from build123d import *

# Parameters (mm, degrees)
EXTRUDE_THIN1_DEPTH = 30
SKETCH2_R           = 4.1
CUT_EXTRUDE1_DEPTH  = 10
BOSS_EXTRUDE1_START = -3
SKETCH3_W           = 40
SKETCH3_H           = 40
BOSS_EXTRUDE1_DEPTH = 15
SKETCH4_R           = 6
BOSS_EXTRUDE2_DEPTH = 5
FILLET1_R           = 2
SKETCH5_W           = 40
SKETCH5_H           = 40
SKETCH5_W_2         = 38
SKETCH5_H_2         = 38
BOSS_EXTRUDE3_DEPTH = 40
SKETCH6_W           = 40
SKETCH6_H           = 40
BOSS_EXTRUDE4_DEPTH = 1
SKETCH7_R           = 2.5
CUT_EXTRUDE2_DEPTH  = 91.691785736


with BuildPart() as part:
    # Sketch1 → Extrude-Thin1 (new body)
    with BuildSketch(Plane(origin=(0, 0, 0), x_dir=(1, 0, 0), z_dir=(0, 1, 0))):
        Polygon((0, 0), (60, 0), (60, -15), (57, -15), (57, -3), (0, -3), align=None)
    extrude(amount=EXTRUDE_THIN1_DEPTH)

    # Sketch2 → Cut-Extrude1 (cut)
    with BuildSketch(Plane.XY.offset(3)):
        with Locations((15, 15)):
            Circle(SKETCH2_R)
    extrude(amount=-CUT_EXTRUDE1_DEPTH, mode=Mode.SUBTRACT)

    # Sketch3 → Boss-Extrude1 (add)
    with BuildSketch(Plane.ZY.offset(-57).offset(BOSS_EXTRUDE1_START)):
        with Locations((35, 20)):
            Rectangle(SKETCH3_W, SKETCH3_H)
    extrude(amount=BOSS_EXTRUDE1_DEPTH)

    # Sketch4 → Boss-Extrude2 (add)
    with BuildSketch(Plane.ZY.offset(-45)):
        with Locations(Location((35, 20, 0), (0, 0, 180))):
            Circle(SKETCH4_R)
    extrude(amount=BOSS_EXTRUDE2_DEPTH)

    # Fillet1
    fillet1_edges = [part.edges().sort_by_distance(p)[0] for p in [
        (45, 20, 41),
    ]]
    fillet(fillet1_edges, radius=FILLET1_R)

    # Sketch5 → Boss-Extrude3 (add)
    with BuildSketch(Plane.ZY.offset(-45)):
        with Locations((35, 20)):
            Rectangle(SKETCH5_W, SKETCH5_H)
        with Locations((35, 20)):
            Rectangle(SKETCH5_W_2, SKETCH5_H_2, mode=Mode.SUBTRACT)
    extrude(amount=BOSS_EXTRUDE3_DEPTH)

    # Sketch6 → Boss-Extrude4 (add)
    with BuildSketch(Plane.ZY.offset(-5)):
        with Locations((35, 20)):
            Rectangle(SKETCH6_W, SKETCH6_H)
    extrude(amount=BOSS_EXTRUDE4_DEPTH)

    # Sketch7 → Cut-Extrude2 (cut, through all)
    with BuildSketch(Plane(origin=(0, 40, 0), x_dir=(1, 0, 0), z_dir=(0, 1, 0))):
        with Locations(Location((15, -35, 0), (0, 0, 270))):
            Circle(SKETCH7_R)
    extrude(amount=-CUT_EXTRUDE2_DEPTH, mode=Mode.SUBTRACT)

    # Sketch8 → Revolve1 (revolve)
    with BuildSketch(Plane.XY.offset(35), mode=Mode.PRIVATE) as revolve1_sk:
        Polygon((17.5, 1), (22.966741001, 8.14945752), (23.966741001, 8.14945752), (23.966741001, 1), align=None)
    revolve(revolve1_sk.sketch.rotate(Axis((15, 1, 35), (0, 1, 0)), 90), axis=Axis((15, 1, 35), (0, 1, 0)))


solid = part.part
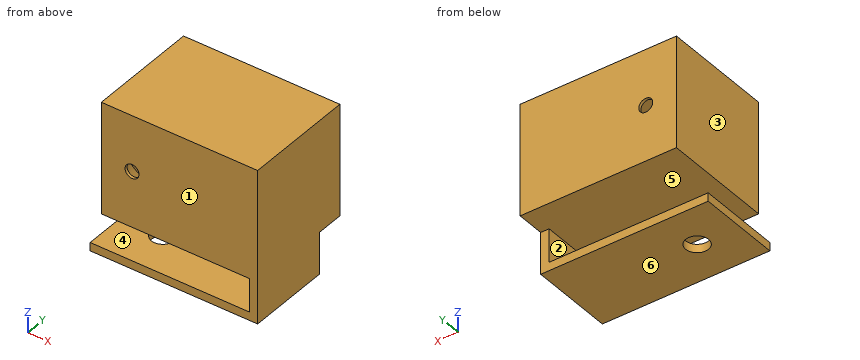
The listing builds one solid part. Answer for the finished solid, in the listing's coordinates (mm). Face numbers are marked on the shaded views. A direction names the side the tool comes from. Give positions to 0.01 mm unless a question says otherwise; leave off trailing zeros. Loops run counter-clockwise (first coordinate to the right, second up) from the corner with the lowest first, then second, coordinate; pieces in that order, holes last. Notation, with made-up numbers: (14.5, -23.5) - (52.5, -23.5) arc R28 ccw to (52.5, 1.5) - close; hole circle Ø10 at (83, -18). An arc over 180 degrees is marked (long way). Use one line per item in the form item = value.
1. Given pin 1 Ø9.5 at (y, z) = (21, 34.5) entering from -X; pin 2 Ø9.5 at (y, z) = (10.5, 8.5) entering from -X; pin 3 Ø7.5 at (x, y) = (15, 15) entering from -Z, each flat-ended and moving along its own axis, determine where each tip first touches the part or whether it passes through.
Calculated:
pin_1 = 4
pin_2 = 57
pin_3 = 15
2. Section B-B on y = 3 is taken. Give the vertices of the cut face in (x, z).
Calculated:
outline = (0, 0) - (60, 0) - (60, 55) - (4, 55) - (4, 15) - (57, 15) - (57, 3) - (0, 3) - close; circle Ø17.93 at (15, 35); hole (5, 16) - (45, 16) - (45, 54) - (5, 54) - close; hole circle Ø8.06 at (15, 35)
3. Section D-D on z = 35 is taken. Give the vertices of the cut face in (x, y), then the cut area to 3 significant figures.
Calculated:
outline = (4, 0) - (12.5, 0) - (12.5, 1) - (7.03, 8.15) - (6.03, 8.15) - (6.03, 1) - (5, 1) - (5, 39) - (12.5, 39) - (12.5, 40) - (4, 40) - close; (17.5, 0) - (60, 0) - (60, 40) - (17.5, 40) - (17.5, 39) - (45, 39) - (45, 28) arc R2 cw to (43, 26) - (40, 26) - (40, 14) - (43, 14) arc R2 cw to (45, 12) - (45, 1) - (23.97, 1) - (23.97, 8.15) - (22.97, 8.15) - (17.5, 1) - close
area = 825 mm^2
4. Section C-C on x = 31 is taken. Give the vertices of the cut face in (y, z).
Calculated:
outline = (0, 0) - (30, 0) - (30, 3) - (0, 3) - close; (0, 15) - (40, 15) - (40, 55) - (0, 55) - close; hole (1, 16) - (39, 16) - (39, 54) - (1, 54) - close
5. Find the intervals of material crossed by line 1 along Z through (x, y) = (5.5, 19.5); line 2 along Y through (x, z) = (9, 51); line 3 along Z through (x, y) = (56, 2.5), in increasing order. Write a range as [from, to].
Calculated:
line_1 = [0, 3], [15, 16], [54, 55]
line_2 = [0, 1], [39, 40]
line_3 = [0, 3], [15, 55]
6. The mould has two halves that part along Z. Classify the marked faces 3, 4, 5 and 6: pulls with the +Z half, pulls with the -Z half, needs draft (parallel to the pull), parting line crosses it, or undercut.
Calculated:
face_3 = needs draft
face_4 = undercut
face_5 = undercut
face_6 = pulls with the -Z half
7. Which of the six approach directions +Z, -Z, +X, -X, +Y, -Y give full straight-line access (tool end or side, diameter ignored) to the marked faces 1 and 2?
Calculated:
face_1 = +Z, -Z, +X, -X, -Y
face_2 = -X, +Y, -Y
8. Section A-A on z = 25 is taken. Give the vertices of the cut face in (x, y), then the cut area to 3 significant figures.
Calculated:
outline = (4, 0) - (60, 0) - (60, 40) - (4, 40) - close; hole (5, 1) - (45, 1) - (45, 39) - (5, 39) - close
area = 720 mm^2
